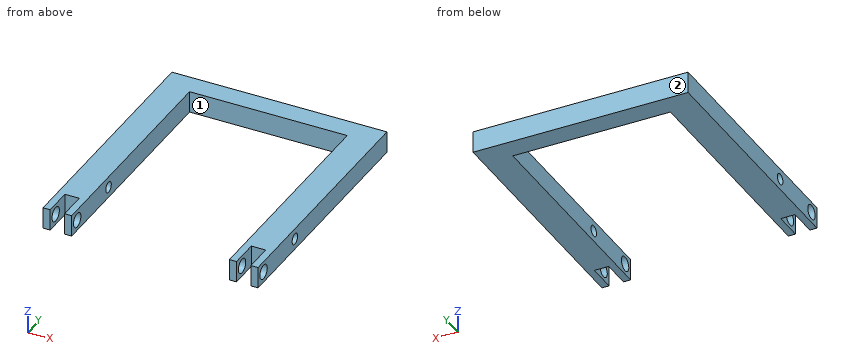
from build123d import *

# Parameters (mm, degrees)
SKETCH2_W           = 300
SKETCH2_H           = 350
BOSS_EXTRUDE1_DEPTH = 30
SKETCH3_W           = 220
SKETCH3_H           = 320
CUT_EXTRUDE1_DEPTH  = 236.67423904
SKETCH4_R           = 7.5
SKETCH4_R_2         = 10
CUT_EXTRUDE2_DEPTH  = 351.773925694
SKETCH7_W           = 20
SKETCH7_H           = 30
CUT_EXTRUDE3_DEPTH  = 40
SKETCH8_W           = 20
SKETCH8_H           = 30
CUT_EXTRUDE4_DEPTH  = 40


with BuildPart() as part:
    # Sketch2 → Boss-Extrude1 (new body)
    with BuildSketch(Plane.XY):
        with Locations((0, 4.282868526)):
            Rectangle(SKETCH2_W, SKETCH2_H)
    extrude(amount=BOSS_EXTRUDE1_DEPTH)

    # Sketch3 → Cut-Extrude1 (cut, through all)
    with BuildSketch(Plane.XY.offset(30)):
        with Locations((0, -10.717131474)):
            Rectangle(SKETCH3_W, SKETCH3_H)
    extrude(amount=-CUT_EXTRUDE1_DEPTH, mode=Mode.SUBTRACT)

    # Sketch4 → Cut-Extrude2 (cut, through all)
    with BuildSketch(Plane.ZY.offset(150)):
        with Locations(Location((15, -70.717131474, 0), (0, 0, 270))):
            Circle(SKETCH4_R)
        with Locations(Location((15, -155.717131474, 0), (0, 0, 270))):
            Circle(SKETCH4_R_2)
    extrude(amount=-CUT_EXTRUDE2_DEPTH, mode=Mode.SUBTRACT)

    # Sketch7 → Cut-Extrude3 (cut)
    with BuildSketch(Plane.XZ.offset(170.717131474)):
        with Locations((-130, 15)):
            Rectangle(SKETCH7_W, SKETCH7_H)
    extrude(amount=-CUT_EXTRUDE3_DEPTH, mode=Mode.SUBTRACT)

    # Sketch8 → Cut-Extrude4 (cut)
    with BuildSketch(Plane.XZ.offset(170.717131474)):
        with Locations((130, 15)):
            Rectangle(SKETCH8_W, SKETCH8_H)
    extrude(amount=-CUT_EXTRUDE4_DEPTH, mode=Mode.SUBTRACT)


solid = part.part
Build history of the part. All positions in model axes, mm. Face numbers are marked on the shaded views. A direction names the side the tool comes from. Coordinates: 2 decimals unless noted, no trailing zeros. Write each loop counter-clockwise with the first axis right and the second up, starting at its lowest first coordinate (ties: lowest second). Pieces come first, ordered by that corner, then holes.
(1) 3-axis set-ups, long thin cutter, end or side, ignore diameter. For the marked faces 1 and 2: which of +Z, -Z, +X, -X, +Y, -Y reach the whole face in a straight line?
(2) Drill centre lines: line 1 (X direction, y = -134.5, z = 19.75); line 2 (X direction, y = -127, z = 18.25); line 3 (Y direction, x = 135, z = 1.5). Where is each one in solid material? Low to high.
(3) Cut at B-B on z = 15. State how many separate pieces and enclosed holes the cut face has, and give its area (3 significant figures).
(4) Cut at C-C on x = 54. List the corners of the cut face in (y, z).
(5) Pin check, flat tips, straight feed: pin 1 Ø10 at (x, z) = (26.5, 23) entering from -Y; pin 2 Ø16 at (y, z) = (-155.72, 15) entering from +X; pin 3 Ø6 at (x, z) = (-131.5, 18) entering from -Y. Stop position of each tip, or through.
(6) Cut at A-A on y = -46. List the corners of the cut face in (x, z).
Working result:
1. face 1: +Z, -Z, -Y
1. face 2: +Z, -Z, +X, -X, +Y
2. line 1: x = -150 to -140, -120 to -110, 110 to 120, 140 to 150
2. line 2: x = -150 to -110, 110 to 150
2. line 3: y = -130.72 to 179.28
3. separate pieces: 7
3. enclosed holes: 0
3. area: 31,000 mm2
4. outline: (149.28, 0) - (179.28, 0) - (179.28, 30) - (149.28, 30) - close
5. pin 1: stops at y = 149.28
5. pin 2: passes through
5. pin 3: stops at y = -130.72
6. outline: (-150, 0) - (-110, 0) - (-110, 30) - (-150, 30) - close; (110, 0) - (150, 0) - (150, 30) - (110, 30) - close
